Build history of the part. All positions in model axes, mm. Round coordinates to 2 decimals unless told otherwise and drop trailing zeros. Loops run counter-clockwise (first coordinate to the right, second up) from the corner with the lowest first, then second, coordinate; pieces in that order, holes last. Notation, with made-up numbers: M 73,56 L 115,56 A21 cw 115,74 Z; hole C 88,-35 d3. An arc over 180 degrees is marked long. One line per item, written item: value.
Autodesk Inventor part; units mm, degrees
ref_plane "YZ Plane" through (0, 0, 0) normal (1, 0, 0) x (0, 1, 0)
ref_plane "XZ Plane" through (0, 0, 0) normal (0, 1, 0) x (-1, 0, 0)
ref_plane "XY Plane" through (0, 0, 0) normal (0, 0, 1) x (1, 0, 0)
sketch "Sketch1" plane through (0, 0, 0) normal (1, 0, 0) x (0, 1, 0)
  line L0 (0, 0) -> (90, 0)
  line L1 (90, 0) -> (90, -70)
  line L2 (90, -70) -> (0, -70)
  line L3 (0, -70) -> (0, 0)
  circle A0 centre (15, -4) radius 1.425
  circle A1 centre (45, -4) radius 1.425
  circle A2 centre (75, -4) radius 1.425
  line L4 (0, -4) -> (90, -4) construction
  line L5 (45, -70) -> (45, 0) construction
  line L6 (0, -35) -> (90, -35) construction
  circle A3 centre (15, -66) radius 1.425
  circle A4 centre (45, -66) radius 1.425
  circle A5 centre (75, -66) radius 1.425
  dimension "d0" = 2.85
  dimension "d1" = 90
  dimension "d2" = 30
  dimension "d3" = 4
  dimension "d4" = 70
extrude "Extrusion1" add sketch "Sketch1" along normal blind 3.2
sketch "Sketch2" plane through (3.2, 0, 0) normal (1, 0, 0) x (0, 0, -1)
  circle A0 centre (66, 75) radius 1.425
  circle A1 centre (4, 75) radius 1.425
  line L0 (70, 90) -> (0, 90)
  line L1 (35, 90) -> (35, -95.4624)
  line L2 (15.06, 84.91) -> (54.94, 84.91)
  line L3 (54.94, 84.91) -> (54.94, 65.09)
  line L4 (54.94, 65.09) -> (15.06, 65.09)
  line L5 (15.06, 65.09) -> (15.06, 84.91)
  line L6 (4, 75) -> (66, 75) construction
  circle A2 centre (11.37, 80.085) radius 1.05
  circle A3 centre (11.37, 69.915) radius 1.05
  circle A4 centre (58.63, 80.085) radius 1.05
  circle A5 centre (58.63, 69.915) radius 1.05
  point P0 (54.94, 75)
  dimension "d7" = 39.88
  dimension "d8" = 19.82
  dimension "d9" = 10.17
  dimension "d10" = 47.26
  dimension "d11" = 2.1
extrude "Extrusion2" cut sketch "Sketch2" against normal through all contours L2 L3 L4 L1 | L1 L4 L5 L2 | A2 | A3 | A4 | A5
fillet "Fillet1" radius 1 4 edges at (1.6, 84.91, -54.94) (1.6, 65.09, -54.94) (1.6, 65.09, -15.06) (1.6, 84.91, -15.06)
properties part number "ServoPlate1"
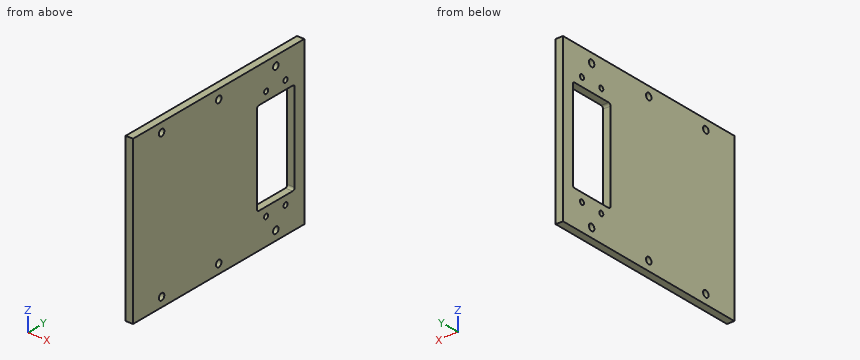
Item 1: Slice it at A-A, the plane y = 15. Give the cut face in (x, z) (3 decimals).
Check values:
outline: M 0,-70 L 3.2,-70 L 3.2,-67.425 L 0,-67.425 Z; M 0,-64.575 L 3.2,-64.575 L 3.2,-5.425 L 0,-5.425 Z; M 0,-2.575 L 3.2,-2.575 L 3.2,0 L 0,0 Z
Item 2: Slice it at B-B, the plane z = -66. Give the cut face in (x, y) (3 decimals), and give its area (3 significant figures).
Check values:
outline: M 0,0 L 3.2,0 L 3.2,13.575 L 0,13.575 Z; M 0,16.425 L 3.2,16.425 L 3.2,43.575 L 0,43.575 Z; M 0,46.425 L 3.2,46.425 L 3.2,73.575 L 0,73.575 Z; M 0,76.425 L 3.2,76.425 L 3.2,90 L 0,90 Z
area: 261 mm2
Item 3: Slice it at D-D, the plane y = 75. Give the cut face in (x, z) (3 decimals), and give its area (3 significant figures).
Check values:
outline: M 0,-70 L 3.2,-70 L 3.2,-67.425 L 0,-67.425 Z; M 0,-64.575 L 3.2,-64.575 L 3.2,-54.94 L 0,-54.94 Z; M 0,-15.06 L 3.2,-15.06 L 3.2,-5.425 L 0,-5.425 Z; M 0,-2.575 L 3.2,-2.575 L 3.2,0 L 0,0 Z
area: 78.1 mm2
Item 4: Slice it at C-C, the plane z = -23.5. Give the cut face in (x, y), and give its area (3 significant figures).
Check values:
outline: M 0,0 L 3.2,0 L 3.2,65.09 L 0,65.09 Z; M 0,84.91 L 3.2,84.91 L 3.2,90 L 0,90 Z
area: 225 mm2
Item 5: Wall check: line 1 along Y through (x, z) = (2.1, -58.63) (3 decimals); line 2 along Y through (x, z) = (0.8, -66) (3 decimals); line 3 along Y through (x, z) = (2.75, -21). Give the ranges that are in metal, low to high.
Check values:
line 1: y = 0 to 68.865, 70.965 to 79.035, 81.135 to 90
line 2: y = 0 to 13.575, 16.425 to 43.575, 46.425 to 73.575, 76.425 to 90
line 3: y = 0 to 65.09, 84.91 to 90
